Part model, mm, in its own coordinate system. A direction names the side the tool comes from. Round coordinates to 2 decimals unless told otherwise and drop trailing zeros. Loops run counter-clockwise (first coordinate to the right, second up) from the corner with the lowest first, then second, coordinate; pieces in that order, holes last.
from build123d import *

# Parameters (mm, degrees)
CHAMFER1_SIZE      = 0.6
CUT_EXTRUDE1_DEPTH = 3


with BuildPart() as part:
    # Sketch1 → Revolve1 (revolve)
    with BuildSketch(Plane.XY, mode=Mode.PRIVATE) as revolve1_sk:
        Polygon((-6, 0), (-6, 5), (0, 5), (0, 3), (60, 3), (60, 0), align=None)
    revolve(revolve1_sk.sketch.rotate(Axis((-6, 0, 0), (1, 0, 0)), 180), axis=Axis((-6, 0, 0), (1, 0, 0)))

    # Chamfer1
    chamfer1_edges = [part.edges().sort_by_distance(p)[0] for p in [
        (-6, 5, 0),
    ]]
    chamfer(chamfer1_edges, length=CHAMFER1_SIZE)

    # Sketch2 → Cut-Revolve1 (revolve, cut)
    with BuildSketch(Plane.XY, mode=Mode.PRIVATE) as cut_revolve1_sk:
        Polygon((-1.497848452, 0), (-3, 2.5), (-6, 2.5), (-6, 0), align=None)
    revolve(cut_revolve1_sk.sketch.rotate(Axis((-6, 0, 0), (1, 0, 0)), 180), axis=Axis((-6, 0, 0), (1, 0, 0)), mode=Mode.SUBTRACT)

    # Sketch3 → Cut-Extrude1 (cut)
    with BuildSketch(Plane.ZY.offset(6)):
        Polygon((0, 2.886751346), (-2.5, 1.443375673), (-2.5, -1.443375673), (0, -2.886751346), (2.5, -1.443375673), (2.5, 1.443375673), align=None)
    extrude(amount=-CUT_EXTRUDE1_DEPTH, mode=Mode.SUBTRACT)


solid = part.part
1) Wall check: line 1 along X through (y, z) = (-3.5, -0.5); line 2 along Z through (x, y) = (52.5, 0); line 3 along Z through (x, y) = (56.5, 2.5). Give the ranges that are in metal, low to high.
Values:
line 1: x = -6 to 0
line 2: z = -3 to 3
line 3: z = -1.66 to 1.66
2) Slice it at A-A, the plane x = 4. Give the cut face in (y, z), then the cut area to 3 significant figures.
Values:
outline: circle Ø6 at (0, 0)
area: 28.3 mm2
3) Drop flat-ended pins along their axis: pin 1 Ø1.4 at (y, z) = (0.5, -1.5) entering from -X; pin 2 Ø2.5 at (x, y) = (-5, 0.5) entering from +Z; pin 3 Ø6 at (x, y) = (22.5, 2.5) entering from +Z; pin 4 Ø1.5 at (x, z) = (24, 0) entering from +Y. Give the stop position or say it passes through.
Values:
pin 1: stops at x = -2.87
pin 2: stops at z = 5
pin 3: stops at z = 3
pin 4: stops at y = 3
4) Mould opens along Z. For faces 3 (the face through (0, -3.3, -0.1)), 4 (the face through (30.42, -2.86, -0.9)), 5 (the face through (-4.521, 2.155, 1.267)) say: released by +Z, released by -Z, zero draft, split by the parting line, or undercut.
Values:
face 3: zero draft
face 4: split by the parting line
face 5: undercut
5) Tool access for faces 1 (the face through (-3, 1.328, -2.295)), 2 (the face through (60, 0, 0)): list every direction of +Z, -Z, +X, -X, +Y, -Y with a clear straight run to the whole face (end or side of a thin tool).
Values:
face 1: -X
face 2: +Z, -Z, +X, +Y, -Y
